from build123d import *

# Parameters (mm, degrees)
F2_R     = 19.05
F3_DEPTH = 25.4
F4_T     = -6.35
F6_D     = 25.4
F6_DEPTH = 82.2327022563
F8_D     = 25.4


with BuildPart() as f1:
    # F0 (on Front) → F1 (revolve)
    with BuildSketch(Plane.XZ):
        Polygon((0, 12.7), (0, 0), (63.1817022563, 0), (63.1817022563, 19.05), align=None)
    revolve(axis=Axis((31.5908511281, 0, 0), (-1, 0, 0)))

    # F2 (on face) → F3 (join)
    with BuildSketch(Plane.YZ.offset(63.1817022563)):
        Circle(F2_R)
    extrude(amount=F3_DEPTH)

    # F4
    f4_openings = [f1.faces().sort_by_distance(p)[0] for p in [
        (88.581702, 0, 0),
    ]]
    offset(amount=F4_T, openings=f4_openings)

    # F6 (through all, one way)
    with BuildSketch(Plane(origin=(6.35, 0, 0), x_dir=(0, 1, 0), z_dir=(-1, 0, 0))):
        with Locations((0, 0)):
            Circle(F6_D / 2)
    extrude(amount=-F6_DEPTH, mode=Mode.SUBTRACT)

    # F8 (through all)
    with Locations(Plane.YZ.offset(6.35)):
        with Locations((0, 0)):
            Hole(F8_D / 2)


solid = f1.part
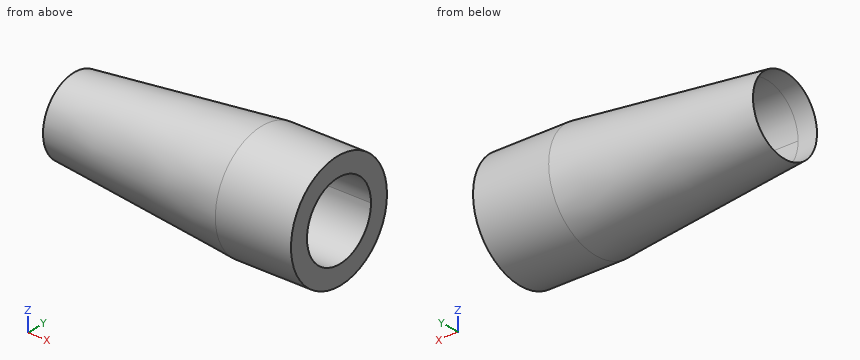
Part model, mm, in its own coordinate system. Coordinates: 2 decimals unless noted, no trailing zeros. Loops run counter-clockwise (first coordinate to the right, second up) from the corner with the lowest first, then second, coordinate; pieces in that order, holes last. Notation, with made-up numbers: M 65.25,13 L 91.25,13 A18 ccw 91.25,18 Z; hole C 85.25,62.25 d4. An arc over 180 degrees is marked long. Use a Markdown table: item, result. Add a question column.
Q1. Cut at C-C (x = 48). Write the cut outline in (y, z), and give its area (3 significant figures).
Q2. Probe L1, parallel to Z at x = 2.25, y = 0; L2, parallel to Z at x = 36, y = 2.5; L3, parallel to Y at x = 28, z = 6.5. List the from-to ranges inside material, lowest first.
Q3. Cut at A-A (y = 0). Write the cut outline in (x, z).
Q4. Pin check, flat tips, straight feed: P1, Ø12, axis at y = 2, z = 13, coming from the -X side; P2, Ø1.5, axis at x = 48.5, z = 3.5, coming from the +Y side; P3, Ø3, axis at x = 66, y = 11, coming from the +Z side; P4, Ø4, axis at x = 66, y = -9.5, coming from the -Z side. Stop position of each tip, or through.
Q5. Cut at B-B (x = 34). Write the cut outline in (y, z), and give its area (3 significant figures).
Worked out:
| question | item | result |
|---|---|---|
| 1 | outline | C 0,0 d35.05; hole C 0,0 d25.4 |
| 1 | area | 458 mm2 |
| 2 | L1 | z = -12.93 to -12.7, 12.7 to 12.93 |
| 2 | L2 | z = -16.13 to -12.45, 12.45 to 16.13 |
| 2 | L3 | y = -14.09 to -10.91, 10.91 to 14.09 |
| 3 | outline | M 0,-12.7 L 63.18,-19.05 L 88.58,-19.05 L 88.58,-12.7 Z; M 0,12.7 L 88.58,12.7 L 88.58,19.05 L 63.18,19.05 Z |
| 4 | P1 | stops at x = 0 |
| 4 | P2 | stops at y = 17.38 |
| 4 | P3 | stops at z = 16.51 |
| 4 | P4 | stops at z = -17.51 |
| 5 | outline | C 0,0 d32.23; hole C 0,0 d25.4 |
| 5 | area | 309 mm2 |
